Can you work these out from the model? Positions are in its coordinate system, mm. A direction names the side the tool comes from. Give positions to 0.01 mm unless a question says otherwise; leave off trailing zeros. Order: outer loops, then holes, each group sorted by start corner. A loop starts at its lowest first (then second) coordinate and runs counter-clockwise, first axis right, second up.
Item 1: If I drill on line 1 along X through (y, z) = (16.5, 4.6); line 2 along X through (y, z) = (5.75, 3); line 3 along X through (y, z) = (4, 0.9), over which ranges is the centre line in solid material (lowest first)?
Item 2: I want a section at C-C, the plane z = 3.1. Write out the boundary of the cut face in (x, y), then the cut area to 3 significant figures.
Item 3: I want a section at B-B, the plane y = 1.5. Write out the boundary of the cut face in (x, z), then the cut area to 3 significant figures.
Item 4: If we mould it in two halves opening along Y, with no side actions, what happens to faces 1 (the flat face through (156, 18, 2)), 2 (the flat face through (3, 5, 2)), 3 (the flat face through (110, 5, 2))? For each: +Y half, -Y half, draft (parallel to the pull), parting line (faces both ways), or undercut.
Item 5: Which directions (+Z, -Z, +X, -X, +Y, -Y) give clear straight access to the entire face, cutting with the end or side of a thin tool? Please do faces 4 (the flat face through (89, 20, 2)), 5 (the flat face through (40, 18, 2)), 6 (the flat face through (171, 10, 2)), 7 (the flat face through (2, 15, 2)), 8 (the flat face through (73.002, 6, 3)).
Item 6: I want a section at A-A, the plane y = 18. Write out the boundary of the cut face in (x, z), then the cut area to 3 significant figures.
Item 7: I'm going to push flat-ended pins straight in: pin 1 Ø1.5 at (y, z) = (11, 2.5) entering from +X; pin 2 Ø0.9 at (y, z) = (6.5, 3.5) entering from -X; pin 3 Ø1.5 at (x, z) = (91, 1.5) entering from -Y. Where does each tip first touch, or does it pass through?
Item 8: I want a section at D-D, the plane x = 90.5. Write out the boundary of the cut face in (y, z).
```python
from build123d import *

# Parameters (mm, degrees)
SALIENTE_EXTRUIR1_DEPTH = 5
CROQUIS2_W              = 30
CROQUIS2_H              = 3
CORTAR_EXTRUIR1_DEPTH   = 10


with BuildPart() as part:
    # Croquis1 → Saliente-Extruir1 (new body)
    with BuildSketch(Plane.XY):
        Polygon((117.333333333, 0), (176, 0), (176, 5), (171, 5), (171, 15), (176, 15), (176, 20), (156, 20), (156, 15), (136, 15), (136, 20), (40, 20), (40, 15), (20, 15), (20, 20), (0, 20), (0, 15), (5, 15), (5, 5), (0, 5), (0, 0), (58.666666667, 0), (58.666666667, 5), (117.333333333, 5), align=None)
    extrude(amount=SALIENTE_EXTRUIR1_DEPTH)

    # Croquis2 → Cortar-Extruir1 (cut)
    with BuildSketch(Plane.XY.offset(5)):
        with Locations((88.001666667, 6.5)):
            Rectangle(CROQUIS2_W, CROQUIS2_H)
    extrude(amount=-CORTAR_EXTRUIR1_DEPTH, mode=Mode.SUBTRACT)


solid = part.part
```
Results list:
1. line 1: x = 0 to 20, 40 to 136, 156 to 176
1. line 2: x = 5 to 73, 103 to 171
1. line 3: x = 0 to 58.67, 117.33 to 176
2. outline: (0, 0) - (58.67, 0) - (58.67, 5) - (73, 5) - (73, 8) - (103, 8) - (103, 5) - (117.33, 5) - (117.33, 0) - (176, 0) - (176, 5) - (171, 5) - (171, 15) - (176, 15) - (176, 20) - (156, 20) - (156, 15) - (136, 15) - (136, 20) - (40, 20) - (40, 15) - (20, 15) - (20, 20) - (0, 20) - (0, 15) - (5, 15) - (5, 5) - (0, 5) - close
2. area: 2,840 mm2
3. outline: (0, 0) - (58.67, 0) - (58.67, 5) - (0, 5) - close; (117.33, 0) - (176, 0) - (176, 5) - (117.33, 5) - close
3. area: 587 mm2
4. face 1: draft
4. face 2: undercut
4. face 3: -Y half
5. face 4: +Z, -Z, +X, -X, +Y
5. face 5: +Z, -Z, +Y
5. face 6: +Z, -Z, +X
5. face 7: +Z, -Z, -X
5. face 8: +Z, -Z, -Y
6. outline: (0, 0) - (20, 0) - (20, 5) - (0, 5) - close; (40, 0) - (136, 0) - (136, 5) - (40, 5) - close; (156, 0) - (176, 0) - (176, 5) - (156, 5) - close
6. area: 680 mm2
7. pin 1: stops at x = 171
7. pin 2: stops at x = 5
7. pin 3: stops at y = 8
8. outline: (8, 0) - (20, 0) - (20, 5) - (8, 5) - close
